```python
from build123d import *

# Parameters (mm, degrees)
BOSS_EXTRUDE1_DEPTH = 0.34
FILLET1_R           = 3
SKETCH3_R           = 23.5
CUT_EXTRUDE1_DEPTH  = 0.5


with BuildPart() as part:
    # Sketch1 → Revolve1 (revolve)
    with BuildSketch(Plane.XY, mode=Mode.PRIVATE) as revolve1_sk:
        Polygon((0, 0), (0, 23), (26.38, 23), (26.38, 19.84), (23.325, 19.84), (21.35, 10.8), (15.5, 9), (15.5, 0), align=None)
    revolve(revolve1_sk.sketch.rotate(Axis((0, 0, 0), (0, 1, 0)), 90), axis=Axis((0, 0, 0), (0, 1, 0)))

    # Sketch2 → Boss-Extrude1 (add)
    with BuildSketch(Plane(origin=(0, 21.75, 0), x_dir=(1, 0, 0), z_dir=(0, 1, 0))):
        with BuildLine():
            ThreePointArc((25.102290732, -25.102290732), (26.38, 0), (25.102290732, 25.102290732))
            ThreePointArc((25.102290732, 25.102290732), (0, 26.38), (-25.102290732, 25.102290732))
            ThreePointArc((-25.102290732, 25.102290732), (-26.38, 0), (-25.102290732, -25.102290732))
            ThreePointArc((-25.102290732, -25.102290732), (0, -26.38), (25.102290732, -25.102290732))
        make_face()
        with BuildLine():
            Line((-19.940411229, 23.122391745), (-19.304015126, 22.485995642))
            ThreePointArc((-19.304015126, 22.485995642), (-19.304015126, 19.304015126), (-22.485995642, 19.304015126))
            Line((-22.485995642, 19.304015126), (-23.122391745, 19.940411229))
            ThreePointArc((-23.122391745, 19.940411229), (-23.122391745, 23.122391745), (-19.940411229, 23.122391745))
        make_face(mode=Mode.SUBTRACT)
        with BuildLine():
            Line((23.122391745, 19.940411229), (22.485995642, 19.304015126))
            ThreePointArc((22.485995642, 19.304015126), (19.304015126, 19.304015126), (19.304015126, 22.485995642))
            Line((19.304015126, 22.485995642), (19.940411229, 23.122391745))
            ThreePointArc((19.940411229, 23.122391745), (23.122391745, 23.122391745), (23.122391745, 19.940411229))
        make_face(mode=Mode.SUBTRACT)
        with BuildLine():
            Line((19.940411229, -23.122391745), (19.304015126, -22.485995642))
            ThreePointArc((19.304015126, -22.485995642), (19.304015126, -19.304015126), (22.485995642, -19.304015126))
            Line((22.485995642, -19.304015126), (23.122391745, -19.940411229))
            ThreePointArc((23.122391745, -19.940411229), (23.122391745, -23.122391745), (19.940411229, -23.122391745))
        make_face(mode=Mode.SUBTRACT)
        with BuildLine():
            Line((-23.122391745, -19.940411229), (-22.485995642, -19.304015126))
            ThreePointArc((-22.485995642, -19.304015126), (-19.304015126, -19.304015126), (-19.304015126, -22.485995642))
            Line((-19.304015126, -22.485995642), (-19.940411229, -23.122391745))
            ThreePointArc((-19.940411229, -23.122391745), (-23.122391745, -23.122391745), (-23.122391745, -19.940411229))
        make_face(mode=Mode.SUBTRACT)
    extrude(amount=-BOSS_EXTRUDE1_DEPTH)

    # Fillet1
    fillet1_edges = [part.edges().sort_by_distance(p)[0] for p in [
        (-25.102290732, 21.58, 25.102290732),
        (-25.102290732, 21.58, -25.102290732),
        (25.102290732, 21.58, -25.102290732),
        (25.102290732, 21.58, 25.102290732),
    ]]
    fillet(fillet1_edges, radius=FILLET1_R)

    # Sketch3 → Cut-Extrude1 (cut)
    with BuildSketch(Plane(origin=(0, 23, 0), x_dir=(1, 0, 0), z_dir=(0, 1, 0))):
        with Locations(Location((0, 0, 0), (0, 0, 270))):
            Circle(SKETCH3_R)
    extrude(amount=-CUT_EXTRUDE1_DEPTH, mode=Mode.SUBTRACT)


solid = part.part
```
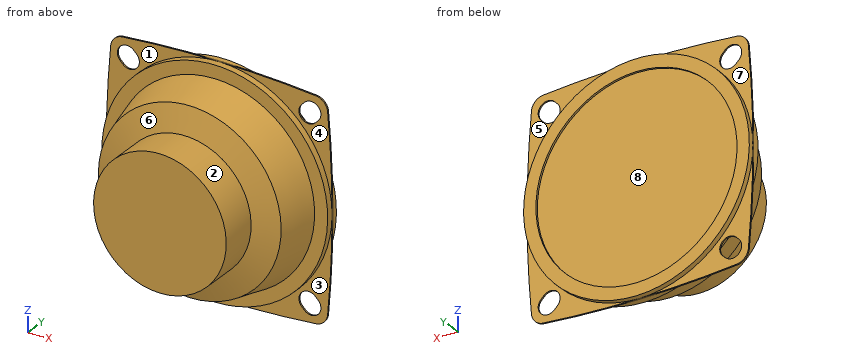
Input: part model. Units: mm. Frame: model coordinates. Face numbers are marked on the shaded views. A direction names the side the tool comes from. Give positions to 0.01 mm unless a question says otherwise; leave off trailing zeros.
1. Material intervals for L1, parallel to X at y = 22.75, z = 0; L2, parallel to Y at x = 19.5, z = 18; L3, parallel to Y at x = -5.5, z = -2, sorted ascending.
Derived:
L1: x = -26.38 to -23.5, 23.5 to 26.38
L2: y = 21.41 to 21.75
L3: y = 0 to 22.5
2. Reachability of the marked faces 1, 2, 3, 4 and 5 from +Z, -Z, +X, -X, +Y, -Y: full face, straight path, thin tool, end or side. Return the list, or none.
Derived:
face 1: +Z, -X, -Y
face 2: -Y
face 3: -Z, +X, -Y
face 4: +Z, +X, -Y
face 5: +Z, +X, +Y
3. Mould query, pull axis Z, two halves, no side actions, for the marked faces 6, 7 and 8. Classes: released by +Z, released by -Z, zero draft, split by the parting line, or undercut.
Derived:
face 6: split by the parting line
face 7: zero draft
face 8: undercut
4. Pin query (flat end, axial travel): pin 1 (10 mm diameter, centred on y = 14, z = 8.5, fed in from -X) (3 decimals); pin 2 (21 mm diameter, centred on x = 11.5, z = -12.5, fed in from -Y); pin 3 (1.5 mm diameter, centred on x = 12.5, y = 8, fed in from +Z); pin 4 (12 mm diameter, centred on x = 14.5, y = 9, fed in from -Z). Return the tip coordinate at first contact, or that it passes through.
Derived:
pin 1: stops at x = -22.275
pin 2: stops at y = 0
pin 3: stops at z = 10.11
pin 4: stops at z = -19.51
